Autodesk Inventor part; units mm, degrees
ref_plane "YZ Plane" through (0, 0, 0) normal (1, 0, 0) x (0, 1, 0)
ref_plane "XZ Plane" through (0, 0, 0) normal (0, 1, 0) x (-1, 0, 0)
ref_plane "XY Plane" through (0, 0, 0) normal (0, 0, 1) x (1, 0, 0)
sketch "Sketch1" plane through (0, 0, 0) normal (0, 0, 1) x (1, 0, 0)
  circle A0 centre (0, 0) radius 1.5
  circle A1 centre (0, 26) radius 1.5
  arc A2 (-4.5, 0) -> (4.5, 0) centre (0, 0) ccw
  line L0 (4.5, 0) -> (4.5, 7.98)
  line L1 (-4.5, 0) -> (-6.4045, 23.6711)
  line L2 (-4.5, 0) -> (21.43, 0) construction
  line L3 (4.5, 7.98) -> (7.7584, 8.7295)
  line L4 (-1.4921, 25.8465) -> (17.6104, 25.8465) construction
  line L5 (-1.372, 54.3276) -> (-2.3083, 54.3276)
  line L6 (-4.5641, 62.9172) -> (-7.4382, 60.7619)
  line L7 (7.7584, 8.7295) -> (4.4705, 26.7439)
  line L8 (-0.0191, 32.9172) -> (4.4705, 26.7439)
  line L9 (0.2933, 53.9165) -> (-1.372, 54.3276)
  line L10 (-4.1293, 46.9816) -> (-4.1293, 41.4235)
  line L11 (-4.1293, 41.4235) -> (-3.8585, 37.8118)
  line L12 (-10.9822, 44.2097) -> (-10.9822, 29.6062)
  line L13 (2.3383, 53.7129) -> (1.6877, 52.735)
  line L14 (-7.4382, 60.7619) -> (-10.9822, 44.2097)
  line L15 (-2.3083, 54.3276) -> (-4.1293, 46.9816)
  line L16 (-6.4045, 23.6711) -> (-10.9822, 29.6062)
  line L17 (-0.0191, 32.9172) -> (-3.8585, 37.8118)
  line L18 (0.3525, 53.9019) -> (1.6877, 52.735)
  line L19 (2.3383, 53.7129) -> (-4.5641, 62.9172)
  line L20 (0.3525, 53.9019) -> (0.2933, 53.9165)
  dimension "d1" = 3
  dimension "d0" = 3
  dimension "d2" = 26
  dimension "d3" = 9
  dimension "d4" = 7.98
  dimension "d6" = 94.6
extrude "Extrusion1" add sketch "Sketch1" along normal blind 3
fillet "Fillet1" radius 10 1 edges at (4.5, 7.98, 1.5)
fillet "Fillet6" radius 11 1 edges at (4.4705, 26.7439, 1.5)
fillet "Fillet7" radius 1.3 1 edges at (2.3383, 53.7129, 1.5)
properties part number "grip1a" material "ABS Plastic"
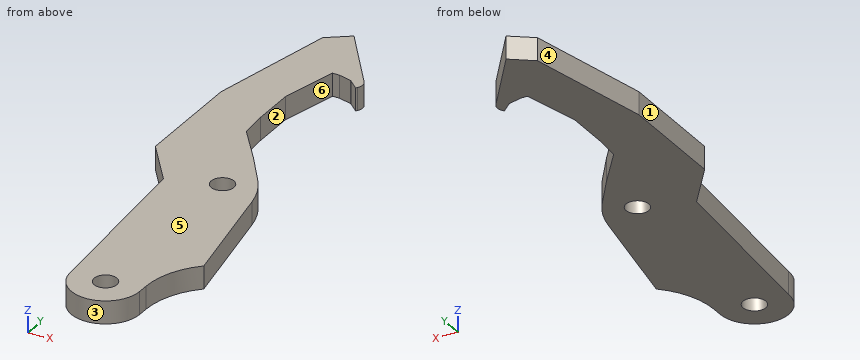
Model file for the job. Use its own axes, mm. Face numbers are marked on the shaded views. A direction names the side the tool comes from. Give positions to 0.01 mm unless a question says otherwise; leave off trailing zeros. Order: outer loops, then holes, each group sorted by start corner. A loop starts at its lowest first (then second) coordinate and runs counter-clockwise, first axis right, second up. Notation, with made-up numbers: (-31, 74) - (-11, 74) arc R26 ccw to (-11, 89) - close; hole circle Ø7 at (70, 12.5). An arc over 180 degrees is marked (long way). Return JSON: item names as keys, results as strings.
1) Flat gauge pins, fed straight in: P1, Ø1.8, axis at x = 0, y = 26, coming from the +Z side; P2, Ø1, axis at x = -1.5, z = 1.5, coming from the -Y side. Where does each tip first touch, or does it go through?
Geometry says:
{"P1": "through", "P2": "y = -4.39"}
2) Cut at D-D, the plane y = 8. Give the cut face in (x, z).
Geometry says:
{"outline": "(-5.14, 0) - (7.04, 0) - (7.04, 3) - (-5.14, 3) - close"}
3) Probe line 1 (Y direction, x = 0, z = 1.6); line 2 (Y direction, x = 0.5, z = 0.8); line 3 (X direction, y = 26.5, z = 1.85). List the from-to ranges inside material, lowest first. Write a range as from..to.
Geometry says:
{"line 1": "-4.5..-1.5, 1.5..24.5, 27.5..32.89, 53.99..56.83", "line 2": "-4.47..-1.41, 1.41..24.59, 27.41..32.2, 53.77..56.16", "line 3": "-8.59..-1.41, 1.41..4.27"}
4) Pull direction Y, two halves, no side cores. Call the marked faces 3, 4, 5 and 6: pulls with the +Y half, pulls with the -Y half, needs draft (parallel to the pull), parting line crosses it, or undercut.
Geometry says:
{"face 3": "pulls with the -Y half", "face 4": "pulls with the +Y half", "face 5": "needs draft", "face 6": "undercut"}
5) Cut at C-C, the plane x = -8.5. Give the cut face in (y, z), plus the area to 3 significant figures.
Geometry says:
{"outline": "(26.39, 0) - (55.8, 0) - (55.8, 3) - (26.39, 3) - close", "area": "88.2 mm²"}
6) Cut at B-B, the plane y = 26. Give the cut face in (x, z).
Geometry says:
{"outline": "(-8.2, 0) - (-1.5, 0) - (-1.5, 3) - (-8.2, 3) - close; (1.5, 0) - (4.46, 0) - (4.46, 3) - (1.5, 3) - close"}
7) 3-axis set-ups, long thin cutter, end or side, ignore diameter. For the marked faces 1 and 2: which of +Z, -Z, +X, -X, +Y, -Y reach the whole face in a straight line?
Geometry says:
{"face 1": "+Z, -Z, -X, +Y, -Y", "face 2": "+Z, -Z, +X"}
8) Cut at A-A, the plane z = 1.4. Count the separate pieces of the cut face and the enclosed holes in it, plus the area to 3 significant figures.
Geometry says:
{"separate pieces": "1", "enclosed holes": "2", "area": "614 mm²"}
